Can you work these out from the model? Positions are in its coordinate system, mm. A direction names the side the tool comes from. Round coordinates to 2 decimals unless told otherwise and drop trailing zeros. Loops run counter-clockwise (first coordinate to the right, second up) from the corner with the lowest first, then second, coordinate; pieces in that order, holes last.
Autodesk Inventor part; units mm, degrees
ref_plane "YZ Plane" through (0, 0, 0) normal (1, 0, 0) x (0, 1, 0)
ref_plane "XZ Plane" through (0, 0, 0) normal (0, 1, 0) x (-1, 0, 0)
ref_plane "XY Plane" through (0, 0, 0) normal (0, 0, 1) x (1, 0, 0)
sketch "Sketch1" plane through (0, 0, 0) normal (0, 0, 1) x (1, 0, 0)
  arc A0 (184.5073, 35.0953) -> (33.1465, 192.9611) centre (-3.7688, 6.072) ccw construction
  arc A1 (184.5073, 35.0953) -> (166.6077, 91.29) centre (-3.7688, 6.072) ccw
  line L0 (202.6605, 59.7837) -> (184.5073, 35.0953)
  arc A2 (202.6605, 59.7837) -> (205.1287, 67.3071) centre (192.4287, 67.3071) ccw
  line L1 (166.6077, 91.29) -> (205.1287, 91.29)
  line L2 (205.1287, 67.3071) -> (205.1287, 91.29)
  point P0 (0, 0)
  dimension "d3" = 12.7
extrude "Extrusion1" add sketch "Sketch1" along normal mid plane 19.05
sketch "Sketch2" plane through (166.6077, 91.29, 9.525) normal (0, 1, 0) x (1, 0, 0)
  circle A0 centre (26.5011, 9.525) radius 3.81
  line L0 (38.5211, 0) -> (38.5211, 19.05) construction
  ellipse E0 centre (26.5011, 5.9613) end of major axis (22.6972, 5.7462) minor radius 3.81 construction
  ellipse E1 centre (26.5011, 5.9613) end of major axis (22.6972, 5.7462) minor radius 3.81 construction
  point P0 (-166.6077, 9.525)
  point P1 (38.5211, 9.525)
  dimension "d6" = 7.62
extrude "Extrusion2" cut sketch "Sketch2" against normal blind 25.4
ref_plane "Work Plane1" through (166.6077, 91.29, 9.525) normal (-0.9528, -0.3035, 0) x (0, 0, -1)
sketch "Sketch3" plane through (166.6077, 91.29, 9.525) normal (-0.9528, -0.3035, 0) x (0, 0, -1)
  circle A0 centre (9.525, 12.7) radius 2.921
  line L0 (0, 0) -> (19.05, 0) construction
  circle A1 centre (9.525, 38.6566) radius 2.921
  line L1 (19.05, 58.9766) -> (0, 58.9766)
  point P0 (9.525, 36.4178)
  point P1 (9.525, 0)
  point P2 (9.525, 0)
  dimension "d9" = 5.842
  dimension "d10" = 12.7
  dimension "d11" = 5.842
  dimension "d12" = 20.32
extrude "Extrusion3" cut sketch "Sketch3" against normal blind 10.16
ref_plane "Work Plane2" through (0, 0, 0) normal (0, 0, 1) x (1, 0, 0)
sketch "Sketch4" plane through (0, 0, 0) normal (0, 0, 1) x (1, 0, 0)
  point P0 (0, 0)
equation "\"d11\" = d9"
properties part number "light_mount"
(1) If we section it at D-D, the plane z = 0: List the corners of the cut face in (x, y) for me, then the cut area to 3 significant figures.
Worked answers:
outline: (166.61, 91.29) arc R190.5 cw to (170.79, 82.36) - (179.26, 85.06) - (181.03, 79.49) - (173.05, 76.95) arc R190.5 cw to (179.54, 57.91) - (187.14, 60.32) - (188.91, 54.76) - (181.05, 52.25) arc R190.5 cw to (184.51, 35.1) - (202.66, 59.78) arc R12.7 ccw to (205.13, 67.31) - (205.13, 91.29) - (196.92, 91.29) - (196.92, 65.89) - (189.3, 65.89) - (189.3, 91.29) - close
area: 989 mm2
(2) If we mould it in two halves opening along X, with no side actions, what happens to faces 1 (the flat face through (180.16, 82.23, 0.04)), 2 (the flat face through (193.7, 47.6, -0.1)), 3 (the flat face through (186, 91.29, 0))? For each: released by +X, released by -X, zero draft, split by the parting line, or undercut.
Worked answers:
face 1: undercut
face 2: released by +X
face 3: zero draft
(3) If we section it at A-A, the plane z = 8: List the corners of the cut face in (x, y) for me, then the cut area to 3 significant figures.
Worked answers:
outline: (166.61, 91.29) arc R190.5 cw to (184.51, 35.1) - (202.66, 59.78) arc R12.7 ccw to (205.13, 67.31) - (205.13, 91.29) - close
area: 1,280 mm2
(4) If we section it at C-C, the plane y = 40.5: List the corners of the cut face in (x, z) for me (3 decimals), then the cut area to 3 significant figures.
Worked answers:
outline: (183.594, -9.525) - (188.481, -9.525) - (188.481, 9.525) - (183.594, 9.525) - close
area: 93.1 mm2
(5) For faces 4 (the flat face through (205.129, 79, 0)), 5 (the flat face through (188.035, 57.502, 0.041)), 6 (the flat face through (193, 65.89, 0)), which set-ups out of +Z, -Z, +X, -X, +Y, -Y let a thin tool reach every point of the face, with its end or its side?
Worked answers:
face 4: +Z, -Z, +X, +Y, -Y
face 5: none
face 6: +Y
(6) Will these pins go through, and if not, where does the flat tip stop? P1, Ø3, axis at y = 77.5, z = 7.5, coming from the -X side; P2, Ø4, axis at x = 201, z = 4, coming from the -Y side; P3, Ø4, axis at x = 192.5, z = 1.5, coming from the +Y side.
Worked answers:
P1: stops at x = 172.22
P2: stops at y = 54.81
P3: stops at y = 65.89
(7) If we section it at B-B, the plane x = 202: List the corners of the cut face in (y, z) for me (3 decimals), then the cut area to 3 significant figures.
Worked answers:
outline: (58.885, -9.525) - (91.29, -9.525) - (91.29, 9.525) - (58.885, 9.525) - close
area: 617 mm2
(8) If I drill on line 1 (Z direction, x = 196, y = 73) (3 decimals); line 2 (X direction, y = 72.25, z = 0); line 3 (X direction, y = 78.5, z = -8.25), over which ranges is the centre line in solid material (lowest first)?
Worked answers:
line 1: z = -9.525 to -2.481, 2.481 to 9.525
line 2: x = 174.87 to 189.3, 196.92 to 205.13
line 3: x = 172.43 to 205.13
